Build history of the part. All positions in model axes, mm. Coordinates: 2 decimals unless noted, no trailing zeros. Loops run counter-clockwise (first coordinate to the right, second up) from the corner with the lowest first, then second, coordinate; pieces in that order, holes last.
(1) Wall check: L1, parallel to Z at x = -131, y = -130.5; L2, parallel to Z at x = 17, y = -78; L3, parallel to Z at x = -24.5, y = -11. Give the ranges that are in metal, low to high.
(2) Slice it at B-B (y = -56.5). Give the cut face in (x, z).
(3) Slice it at D-D (y = -24). Give the cut face in (x, z).
(4) Flat gauge pins, fed straight in: P1, Ø6, axis at x = -52.5, y = -82.5, coming from the +Z side; P2, Ø3, axis at x = 32.5, y = -14, coming from the +Z side; P3, Ø8, axis at x = 31, z = 117, coming from the +Y side. Where does each tip first touch, or does it go through?
(5) Two-plate mould, pull along Z, no slides. Class faces 1 (the face through (3, -69, 88.9)), 2 (the face through (2.934, -89.617, 139.405)), 3 (the face through (209.55, -71, 54)), 4 (the face through (2.93, -90.65, 137.8)): pulls with the +Z half, pulls with the -Z half, needs draft (parallel to the pull), parting line crosses it, or undercut.
(6) Slice it at C-C (x = 59). Give the cut face in (y, z), and give its area (3 significant figures).
(7) Slice it at A-A (x = 144.5). Give the cut face in (y, z), and give its area (3 significant figures).
from build123d import *

# Parameters (mm, degrees)
F1_DEPTH = 209.55
F2_W     = 51.59375
F2_H     = 12.7
F3_DEPTH = 0.4064


# Not quite as in the source:
# - the dataset's text gives a spline's control points without its knots; the knots are read off the source's solid


with BuildPart() as f1:
    # F0 (on Right) → F1 (new body, symmetric)
    with BuildSketch(Plane.YZ):
        Polygon((-139.7, 0), (0, 0), (0, 88.9), (-139.2936, 88.9), (-139.2936, 89.154), (-40.6298144724, 187.8177855276), (-40.9171826682, 188.1051537235), (-139.7, 89.3223363917), align=None)
    extrude(amount=F1_DEPTH, both=True)

    # F2 (on face) → F3 (cut, through all)
    with BuildSketch(Plane(origin=(0, -114.5111681959, 114.5111681959), x_dir=(1, 0, 0), z_dir=(0, -0.7071067812, 0.7071067812))):
        with Locations((133.3471488731, 34.6446699547)):
            Rectangle(F2_W, F2_H)
        with BuildLine():
            add(Edge.make_bspline(
                [(29.4310752731, 11.2932815547), (26.7125386731, 14.0114625547), (22.8919722731, 15.5939587547), (19.0471996731, 15.5939587547)],
                knots=[7, 7, 7, 7, 8, 8, 8, 8], degree=3))
            add(Edge.make_bspline(
                [(19.0471996731, 15.5939587547), (15.2031636731, 15.5939587547), (11.3825972731, 14.0114625547), (8.6636796731, 11.2932815547)],
                knots=[0, 0, 0, 0, 1, 1, 1, 1], degree=3))
            add(Edge.make_bspline(
                [(8.6636796731, 11.2932815547), (5.9454986731, 8.5747703547), (4.3628246731, 4.7539753547), (4.3628246731, 0.9095837547), (4.3628246731, -2.9346046453), (5.9454986731, -6.7553996453), (8.6636796731, -9.4735806453)],
                knots=[1, 1, 1, 1, 2, 2, 2, 3, 3, 3, 3], degree=3))
            add(Edge.make_bspline(
                [(8.6636796731, -9.4735806453), (11.3825972731, -12.1920918453), (15.2031636731, -13.7747912453), (19.0471996731, -13.7747912453), (22.8919722731, -13.7747912453), (26.7125386731, -12.1920918453), (29.4310752731, -9.4735806453), (32.1492816731, -6.7553996453), (33.7315746731, -2.9346046453), (33.7315746731, 0.9095837547), (33.7315746731, 4.7539753547), (32.1492816731, 8.5747703547), (29.4310752731, 11.2932815547)],
                knots=[3, 3, 3, 3, 4, 4, 4, 5, 5, 5, 6, 6, 6, 7, 7, 7, 7], degree=3))
        make_face()
    extrude(amount=-F3_DEPTH, mode=Mode.SUBTRACT)


solid = f1.part
Response values:
1. L1: z = 0 to 88.9, 97.95 to 98.52
1. L2: z = 0 to 88.9, 150.45 to 151.02
1. L3: z = 0 to 88.9
2. outline: (-209.55, 0) - (209.55, 0) - (209.55, 88.9) - (-209.55, 88.9) - close; (-209.55, 171.95) - (209.55, 171.95) - (209.55, 172.52) - (-209.55, 172.52) - close
3. outline: (-209.55, 0) - (209.55, 0) - (209.55, 88.9) - (-209.55, 88.9) - close
4. P1: stops at z = 149.52
4. P2: stops at z = 88.9
4. P3: stops at y = -107.45
5. face 1: undercut
5. face 2: pulls with the +Z half
5. face 3: needs draft
5. face 4: undercut
6. outline: (-139.7, 0) - (0, 0) - (0, 88.9) - (-139.29, 88.9) - (-139.29, 89.15) - (-40.63, 187.82) - (-40.92, 188.11) - (-139.7, 89.32) - close
6. area: 12,500 mm2
7. outline: (-139.7, 0) - (0, 0) - (0, 88.9) - (-139.29, 88.9) - (-139.29, 89.15) - (-94.22, 134.23) - (-94.5, 134.52) - (-139.7, 89.32) - close; (-85.52, 143.5) - (-85.24, 143.21) - (-40.63, 187.82) - (-40.92, 188.11) - close
7. area: 12,500 mm2
